CAD build for the part. Positions are in the model's coordinates, mm. Face numbers are marked on the shaded views. A direction names the side the tool comes from. Round coordinates to 2 decimals unless told otherwise and drop trailing zeros. Write each loop counter-clockwise with the first axis right and the second up, starting at its lowest first coordinate (ties: lowest second). Pieces come first, ordered by that corner, then holes. Notation, with made-up numbers: (82.5, -23.75) -> (106.5, -23.75) arc R23 cw to (106.5, 2.25) -> close; hole circle Ø2 at (9.5, -39). An arc over 180 degrees is marked (long way). Answer in a Markdown table with one row per item. Add a question column.
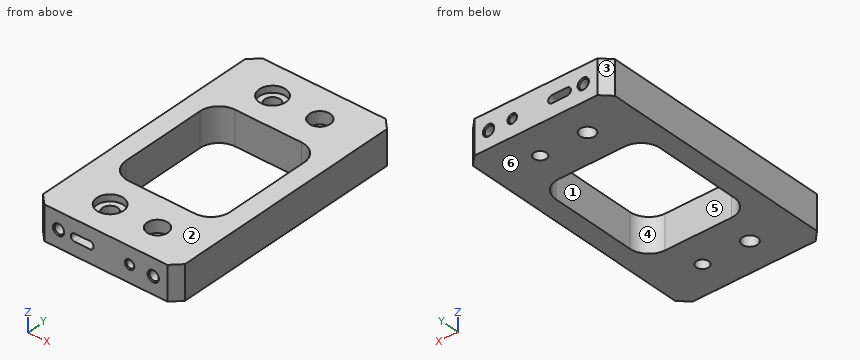
Autodesk Inventor part; units mm, degrees
ref_plane "YZ Plane" through (0, 0, 0) normal (1, 0, 0) x (0, 1, 0)
ref_plane "XZ Plane" through (0, 0, 0) normal (0, 1, 0) x (-1, 0, 0)
ref_plane "XY Plane" through (0, 0, 0) normal (0, 0, 1) x (1, 0, 0)
sketch "3H7Slot" plane through (0, 0, 0) normal (0, 0, 1) x (1, 0, 0)
  line L0 (32.4992, 25.6932) -> (32.4992, 24.1932) construction
  line L1 (30.9992, 25.6932) -> (30.9992, 24.1932)
  line L2 (33.9992, 24.1932) -> (33.9992, 25.6932)
  arc A0 (33.9992, 25.6932) -> (30.9992, 25.6932) centre (32.4992, 25.6932) ccw
  arc A1 (30.9992, 24.1932) -> (33.9992, 24.1932) centre (32.4992, 24.1932) ccw
  point P0 (32.4992, 24.6932)
  dimension "d61" = 3
  dimension "d71" = 1.5
sketch "Sketch1" plane through (32.5, -67.2, -9) normal (0, 0, -1) x (-1, 0, 0)
  point P0 (32.5, 67.2)
sketch "Sketch2" plane through (-32.5, -67.2, 9) normal (0, 0, 1) x (1, 0, 0)
  line L0 (-5, 129.4) -> (-5, 5)
  line L1 (-5, 5) -> (0, 0)
  line L2 (0, 0) -> (65, 0)
  line L3 (65, 0) -> (70, 5)
  line L4 (70, 129.4) -> (70, 5)
  line L5 (70, 129.4) -> (65, 134.4)
  line L6 (0, 134.4) -> (65, 134.4)
  line L7 (0, 134.4) -> (-5, 129.4)
  line L8 (15, 34.4) -> (50, 34.4)
  arc A0 (5, 44.4) -> (15, 34.4) centre (15, 44.4) ccw
  line L9 (5, 90) -> (5, 44.4)
  arc A1 (15, 100) -> (5, 90) centre (15, 90) ccw
  line L10 (50, 100) -> (15, 100)
  arc A2 (60, 90) -> (50, 100) centre (50, 90) ccw
  line L11 (60, 44.4) -> (60, 90)
  arc A3 (50, 34.4) -> (60, 44.4) centre (50, 44.4) ccw
  circle A4 centre (20, 17.2) radius 5.5
  circle A5 centre (45, 17.2) radius 5.5
  circle A6 centre (45, 117.2) radius 5.5
  circle A7 centre (20, 117.2) radius 5.5
  circle A8 centre (32.497, 129.748) radius 2
  arc A9 (34.497, 121.251) -> (30.497, 121.251) centre (32.497, 121.251) ccw
  line L12 (30.497, 113.251) -> (30.497, 121.251)
  arc A10 (30.497, 113.251) -> (34.497, 113.251) centre (32.497, 113.251) ccw
  line L13 (34.497, 121.251) -> (34.497, 113.251)
  point P0 (32.5, 67.2)
sketch "Sketch3" plane through (-32.5, 67.2, -9) normal (0, 1, 0) x (1, 0, 0)
  line L0 (65, 0) -> (0, 0)
  line L1 (0, 0) -> (0, -18)
  line L2 (0, -18) -> (65, -18)
  line L3 (65, -18) -> (65, 0)
  circle A0 centre (7.5, -9) radius 3.5
  circle A1 centre (57.5, -9) radius 3.5
  arc A2 (24, -11) -> (24, -7) centre (24, -9) ccw
  line L4 (16, -11) -> (24, -11)
  arc A3 (16, -7) -> (16, -11) centre (16, -9) ccw
  line L5 (24, -7) -> (16, -7)
  circle A4 centre (45, -9) radius 2
  point P0 (32.5, -9)
sketch "Sketch4" plane through (-32.5, -67.2, 9) normal (0, -1, 0) x (1, 0, 0)
  line L0 (0, 0) -> (65, 0)
  line L1 (0, 0) -> (0, -18)
  line L2 (65, -18) -> (0, -18)
  line L3 (65, -18) -> (65, 0)
  circle A0 centre (45, -9) radius 2
  line L4 (16, -11) -> (24, -11)
  arc A1 (16, -7) -> (16, -11) centre (16, -9) ccw
  line L5 (24, -7) -> (16, -7)
  arc A2 (24, -11) -> (24, -7) centre (24, -9) ccw
  circle A3 centre (57.5, -9) radius 3.5
  circle A4 centre (7.5, -9) radius 3.5
  point P0 (32.5, -9)
extrude "Extrusion1" add sketch "Sketch2" against normal up to surface (18 mm away) from surface at 0 contours L7 L6 L5 L4 L3 L2 L1 L0 | A4 | A5 | A6 | A7 | A8 | L13 A10 L12 A9
hole "M6Clearance" at (12.5, -50, 9) at (12.5, 50, 9) direction (0, 0, -1) diameter 6.6 end through all counterbore diameter 11 counterbore depth 6.5
hole "M6TapsTop" at (25, 67.2, 0) at (-25, 67.2, 0) direction (0, -1, 0) diameter 4.917 depth 17.1 tip angle 118 countersink diameter 6 countersink angle 90
hole "M6TapsBottom" at (25, -67.2, 0) at (-25, -67.2, 0) direction (0, 1, 0) diameter 4.917 depth 17.1 tip angle 118 countersink diameter 6 countersink angle 90
extrude "4H7AlignmentSlot1" cut sketch "Sketch3" against normal blind 8 contours L4 A3 L5 A2
extrude "4H7AlignmentSlot2" cut sketch "Sketch4" against normal blind 8 contours A1 L5 A2 L4
hole "4H7AlignmentHole1" at (12.5, -67.2, 0) direction (0, 1, 0) diameter 4 depth 8 tip angle 118 countersink diameter 5 countersink angle 90
hole "4H7AlignmentHole2" at (12.5, 67.2, 0) direction (0, -1, 0) diameter 4 depth 8 tip angle 118 countersink diameter 5 countersink angle 90
hole "ShoulderScrewHoles" at (-12.5, 50, 9) at (-12.5, -50, 9) direction (0, 0, -1) diameter 8 end through all counterbore diameter 14 counterbore depth 3.5
properties part number "FAB-P0003" material "SolidWorks Materials|6061-T6 (SS)"
Item 1: Two-plate mould, pull along Y, no slides. Class the marked faces 1, 2, 3 and 4: +Y half, -Y half, draft (parallel to the pull), parting line (faces both ways), or undercut.
Item 2: Pin check, flat tips, straight feed: pin 1 (3 mm diameter, centred on x = 25, z = 0, fed in from +Y); pin 2 (3 mm diameter, centred on x = 12.5, z = 0, fed in from -Y); pin 3 (6 mm diameter, centred on x = 12.5, y = -50, fed in from +Z); pin 4 (13 mm diameter, centred on x = -12.5, y = 50, fed in from +Z). Stop position of each tip, or through.
Item 3: Saw through at B-B on y = 12.5. Give the cut face in (x, z).
Item 4: Drill centre lines: probe 1 along X at (y, z) = (50, -3.5); probe 2 along Y at (x, z) = (12.5, -4.5); probe 3 along Y at (x, z) = (-12.5, 2.25). Where is each one in solid material? Low to high.
Item 5: Tool access for the marked faces 5 and 6: list every direction of +Z, -Z, +X, -X, +Y, -Y with a clear straight run to the whole face (end or side of a thin tool).
Item 6: Saw through at A-A on z = 7.5. Give the cut face in (x, y), then the cut area to 3 significant figures.
Item 7: Saw through at D-D on z = -6.75. Give the cut face in (x, y), then the cut area to 3 significant figures.
Item 8: Saw through at C-C on x = -10.5. Count the separate pieces of the cut face and the enclosed holes in it, then the cut area to 3 significant figures.
Recorded:
| question | item | result |
|---|---|---|
| 1 | face 1 | undercut |
| 1 | face 2 | draft |
| 1 | face 3 | +Y half |
| 1 | face 4 | undercut |
| 2 | pin 1 | y = 49.52 |
| 2 | pin 2 | y = -58.9 |
| 2 | pin 3 | through |
| 2 | pin 4 | z = 5.5 |
| 3 | outline | (-37.5, -9) -> (-27.5, -9) -> (-27.5, 9) -> (-37.5, 9) -> close; (27.5, -9) -> (37.5, -9) -> (37.5, 9) -> (27.5, 9) -> close |
| 4 | probe 1 | -37.5 to -16.5, -8.5 to 9.2, 15.8 to 37.5 |
| 4 | probe 2 | -67.2 to -53.3, -46.7 to -32.8, 32.8 to 46.7, 53.3 to 67.2 |
| 4 | probe 3 | -67.2 to -54, -46 to -32.8, 32.8 to 46, 54 to 67.2 |
| 5 | face 5 | +Z, -Z |
| 5 | face 6 | -Z, +X, -X, +Y, -Y |
| 6 | outline | (-37.5, -62.2) -> (-32.5, -67.2) -> (32.5, -67.2) -> (37.5, -62.2) -> (37.5, 62.2) -> (32.5, 67.2) -> (-32.5, 67.2) -> (-37.5, 62.2) -> close; hole (-27.5, -22.8) arc R10 ccw to (-17.5, -32.8) -> (17.5, -32.8) arc R10 ccw to (27.5, -22.8) -> (27.5, 22.8) arc R10 ccw to (17.5, 32.8) -> (-17.5, 32.8) arc R10 ccw to (-27.5, 22.8) -> close; hole circle Ø14 at (-12.5, -50); hole circle Ø14 at (-12.5, 50); hole circle Ø11 at (12.5, -50); hole circle Ø11 at (12.5, 50) |
| 6 | area | 6,010 mm2 |
| 7 | outline | (-37.5, -62.2) -> (-32.5, -67.2) -> (32.5, -67.2) -> (37.5, -62.2) -> (37.5, 62.2) -> (32.5, 67.2) -> (-32.5, 67.2) -> (-37.5, 62.2) -> close; hole (-27.5, -22.8) arc R10 ccw to (-17.5, -32.8) -> (17.5, -32.8) arc R10 ccw to (27.5, -22.8) -> (27.5, 22.8) arc R10 ccw to (17.5, 32.8) -> (-17.5, 32.8) arc R10 ccw to (-27.5, 22.8) -> close; hole circle Ø8 at (-12.5, -50); hole circle Ø8 at (-12.5, 50); hole circle Ø6.6 at (12.5, -50); hole circle Ø6.6 at (12.5, 50) |
| 7 | area | 6,340 mm2 |
| 8 | separate pieces | 4 |
| 8 | enclosed holes | 0 |
| 8 | area | 880 mm2 |
